Verification items for the finished model (mm, model axes). A direction names the side the tool comes from. Give positions to 0.01 mm unless a question says otherwise; leave off trailing zeros. Loops run counter-clockwise (first coordinate to the right, second up) from the corner with the lowest first, then second, coordinate; pieces in that order, holes last. Notation, with made-up numbers: (5, 31) - (37, 31) arc R16 ccw to (37, 37) - close; hole circle Ø5 at (33, -10.75). An arc over 180 degrees is marked (long way). Put each result on its own line as item: value. Start each with the question number.
Autodesk Inventor part; units mm, degrees
ref_plane "YZ Plane" through (0, 0, 0) normal (1, 0, 0) x (0, 1, 0)
ref_plane "XZ Plane" through (0, 0, 0) normal (0, 1, 0) x (-1, 0, 0)
ref_plane "XY Plane" through (0, 0, 0) normal (0, 0, 1) x (1, 0, 0)
sketch "Sketch1" plane through (0, 0, 0) normal (0, 0, 1) x (1, 0, 0)
  line L0 (-57.23, 25.5) -> (57.23, 25.5)
  line L1 (57.23, 25.5) -> (57.23, -25.48)
  line L2 (57.23, -25.48) -> (-57.23, -25.48)
  line L3 (-57.23, -25.48) -> (-57.23, 25.5)
  line L4 (-42.25, 19) -> (42.25, 19)
  line L5 (50, 11.3) -> (50, -13.2)
  line L6 (-50, -13.2) -> (-50, 11.3)
  line L7 (-53.6456, 17.3) -> (53.2492, 17.3) construction
  line L8 (-53.6456, -19.2) -> (53.2492, -19.2) construction
  line L9 (48.25, -31.9957) -> (48.25, 43.3545) construction
  line L10 (-48.25, 39.0692) -> (-48.25, -34.8525) construction
  line L11 (48.25, -15.2) -> (48, -15.2)
  line L12 (48.25, 13.3) -> (48, 13.3)
  line L13 (44.25, 17.3) -> (44.25, 17)
  line L14 (-48.25, 13.3) -> (-48, 13.3)
  line L15 (-44.25, 17.3) -> (-44.25, 17)
  line L16 (-48.25, -15.2) -> (-48, -15.2)
  arc A0 (-50, -13.2) -> (-48, -15.2) centre (-48, -13.2) ccw
  arc A1 (-48, 13.3) -> (-50, 11.3) centre (-48, 11.3) ccw
  arc A2 (-42.25, 19) -> (-44.25, 17) centre (-42.25, 17) ccw
  arc A3 (44.25, 17) -> (42.25, 19) centre (42.25, 17) ccw
  arc A4 (50, 11.3) -> (48, 13.3) centre (48, 11.3) ccw
  arc A5 (48, -15.2) -> (50, -13.2) centre (48, -13.2) ccw
  arc A6 (52.25, 17.3) -> (48.25, 21.3) centre (48.25, 17.3) ccw
  arc A7 (44.25, 17.3) -> (48.25, 13.3) centre (48.25, 17.3) ccw
  arc A8 (48.25, -15.2) -> (44.25, -19.2) centre (48.25, -19.2) ccw
  arc A9 (48.25, -23.2) -> (52.25, -19.2) centre (48.25, -19.2) ccw
  line L17 (50, -19) -> (48.25, -19)
  arc A10 (-48.25, 13.3) -> (-44.25, 17.3) centre (-48.25, 17.3) ccw
  arc A11 (-48.25, 21.3) -> (-52.25, 17.3) centre (-48.25, 17.3) ccw
  arc A12 (-44.25, -19.2) -> (-48.25, -15.2) centre (-48.25, -19.2) ccw
  arc A13 (-52.25, -19.2) -> (-48.25, -23.2) centre (-48.25, -19.2) ccw
  line L18 (44.255, -19) -> (-44.255, -19)
  line L19 (-48.25, -19) -> (-50, -19)
  point P0 (0, 0)
  point P1 (-50, 19)
  point P2 (50, 19)
  point P3 (-50, 13.3)
  point P4 (-50, -15.2)
  dimension "d0" = 114.46
  dimension "d1" = 57.23
  dimension "d2" = 25.5
  dimension "d3" = 25.48
  dimension "d4" = 100
  dimension "d10" = 50
  dimension "d11" = 17.3
  dimension "d12" = 19.2
  dimension "d13" = 96.5
  dimension "d14" = 48.25
  dimension "d19" = 2
  dimension "d20" = 2
extrude "Extrusion1" add sketch "Sketch1" along normal blind 4
sketch "Sketch2" plane through (0, 0, 0) normal (0, 0, -1) x (-1, 0, 0)
  line L0 (57.23, -25.48) -> (57.23, 25.5)
  line L1 (57.23, -25.48) -> (-57.23, -25.48)
  line L2 (57.23, 25.5) -> (-57.23, 25.5)
  line L3 (-57.23, 25.5) -> (-57.23, -25.48)
  line L4 (-57.23, -25.48) -> (57.23, -25.48)
  line L5 (57.23, -25.48) -> (57.23, 25.5)
  line L6 (53.885, 22.255) -> (-53.885, 22.255)
  line L7 (-53.885, 22.255) -> (-53.885, -22.255)
  line L8 (-53.885, -22.255) -> (53.885, -22.255)
  line L9 (53.885, -22.255) -> (53.885, 22.255)
  line L10 (-53.885, 5.805) -> (-51.735, 5.805)
  line L11 (-51.735, 5.805) -> (-51.735, -5.805)
  line L12 (-51.735, -5.805) -> (-53.885, -5.805)
  line L13 (-53.885, -5.805) -> (-53.885, 5.805)
  line L14 (53.885, 5.805) -> (51.735, 5.805)
  line L15 (51.735, 5.805) -> (51.735, -5.805)
  line L16 (51.735, -5.805) -> (53.885, -5.805)
  line L17 (53.885, -5.805) -> (53.885, 5.805)
  line L18 (-51.735, 4.5637) -> (-53.885, 5.805)
  line L19 (-51.735, -4.5637) -> (-53.885, -5.805)
  line L20 (51.735, 4.5637) -> (53.885, 5.805)
  line L21 (51.735, -4.5637) -> (53.885, -5.805)
  point P0 (0, 0)
  dimension "d23" = 44.51
  dimension "d24" = 22.255
  dimension "d25" = 107.77
  dimension "d26" = 53.885
  dimension "d28" = 103.47
  dimension "d30" = 51.735
  dimension "d31" = 11.61
  dimension "d32" = 5.805
  dimension "d33" = 11.61
  dimension "d34" = 5.805
  dimension "d35" = 30
  dimension "d36" = 30
  dimension "d37" = 30
  dimension "d38" = 30
extrude "Extrusion2" add sketch "Sketch2" along normal blind 21 contours L1 L3 L2 L0 | L9 L21 L15 L20 | L18 L11 L19 L7
fillet "Fillet1" radius 6 4 edges at (57.23, 25.5, -8.5) (-57.23, 25.5, -8.5) (57.23, -25.48, -8.5) (-57.23, -25.48, -8.5)
fillet "Fillet2" radius 2 8 edges at (0, -25.48, 4) (55.4726, -23.7226, 4) (57.23, 0.01, 4) (55.4726, 23.7426, 4) (0, 25.5, 4) (-55.4726, 23.7426, 4) (-57.23, 0.01, 4) (-55.4726, -23.7226, 4)
properties part number "EC3BK-40mm_Case_EndCap"
1) Section check B-B, the plane x = -33. Enter the section's corners in (y, z) (3 decimals).
2) Scan lines: line 1 along Y through (x, z) = (-4.5, -1.25) (3 decimals); line 2 along X through (y, z) = (-7, 1.5); line 3 along X through (y, z) = (-9.5, -13.25) (3 decimals). Record each from-to range of solid material in increasing order. Write a range as from..to.
3) Section check A-A, the plane y = -3. Enter the section's corners in (x, z) (3 decimals), plus the area to 3 significant figures.
4) Set-up check for faces 1 (the face through (57.23, 0, -10)), 2 (the face through (50, -1, 2)), 3 (the face through (1, -22.255, -10)): record each of +Z, -Z, +X, -X, +Y, -Y from which the full face is reachable in a straight line by a thin tool's end or side.
5) Section check C-C, the plane z = -8.25. Enter the section's corners in (x, y) (3 decimals).
6) Draft check along X on faces 4 (the face through (0, 20, 0)), 5 (the face through (-57.23, 0, -10)), 6 (the face through (-0.72, -24.91, 3.4)). Enter one of: pulls with the +X half, pulls with the -X half, needs draft (parallel to the pull), parting line crosses it, or undercut.
Results are:
1. outline: (-25.48, -21) - (-22.255, -21) - (-22.255, 0) - (-19, 0) - (-19, 4) - (-23.48, 4) arc R2 ccw to (-25.48, 2) - close; (19, 0) - (22.255, 0) - (22.255, -21) - (25.5, -21) - (25.5, 2) arc R2 ccw to (23.5, 4) - (19, 4) - close
2. line 1: y = -25.48..-22.255, 22.255..25.5
2. line 2: x = -57.23..-50, 50..57.23
2. line 3: x = -57.23..-53.885, 53.885..57.23
3. outline: (-57.23, -21) - (-51.735, -21) - (-51.735, 0) - (-50, 0) - (-50, 4) - (-55.23, 4) arc R2 ccw to (-57.23, 2) - close; (50, 0) - (51.735, 0) - (51.735, -21) - (57.23, -21) - (57.23, 2) arc R2 ccw to (55.23, 4) - (50, 4) - close
3. area: 287 mm2
4. face 1: +Z, -Z, +X, +Y, -Y
4. face 2: +Z, -Z
4. face 3: -Z
5. outline: (-57.23, -19.48) arc R6 ccw to (-51.23, -25.48) - (51.23, -25.48) arc R6 ccw to (57.23, -19.48) - (57.23, 19.5) arc R6 ccw to (51.23, 25.5) - (-51.23, 25.5) arc R6 ccw to (-57.23, 19.5) - close; hole (-53.885, -22.255) - (53.885, -22.255) - (53.885, -5.805) - (51.735, -4.564) - (51.735, 4.564) - (53.885, 5.805) - (53.885, 22.255) - (-53.885, 22.255) - (-53.885, 5.805) - (-51.735, 4.564) - (-51.735, -4.564) - (-53.885, -5.805) - close
6. face 4: undercut
6. face 5: pulls with the -X half
6. face 6: needs draft
